from build123d import *

# Parameters (mm, degrees)
F0_R          = 28.5
F0_R_2        = 26.5
F1_DEPTH      = 1800
F2_R          = 5.25
F2_R_2        = 6
F3_DEPTH      = 28.501
F3_DEPTH_BACK = 28.501
F6_DEPTH      = 5
F7_R          = 5
F8_DEPTH      = 70
F11_DEPTH     = 5
F14_DEPTH     = 5


with BuildPart() as f1:
    # F0 (on Top) → F1 (new body)
    with BuildSketch(Plane.XY):
        Circle(F0_R)
        Circle(F0_R_2, mode=Mode.SUBTRACT)
    extrude(amount=F1_DEPTH)

    # F2 (on Front) → F3 (cut, two sides)
    with BuildSketch(Plane.XZ) as f3_sk:
        with Locations((0, 50)):
            Circle(F2_R)
        with Locations((0, 150)):
            Circle(F2_R)
        with Locations((0, 1420)):
            Circle(F2_R_2)
    extrude(amount=-F3_DEPTH, mode=Mode.SUBTRACT)
    extrude(f3_sk.sketch, amount=F3_DEPTH_BACK, mode=Mode.SUBTRACT)

    # F5 (on offset) → F6 (join)
    with BuildSketch(Plane.XZ.offset(28)):
        Polygon((-5, 41.3397459622), (5, 41.3397459622), (10, 50), (5, 58.6602540378), (-5, 58.6602540378), (-10, 50), align=None)
        Polygon((-5, 141.3397459622), (5, 141.3397459622), (10, 150), (5, 158.6602540378), (-5, 158.6602540378), (-10, 150), align=None)
    extrude(amount=F6_DEPTH)

    # F7 (on offset) → F8 (join)
    with BuildSketch(Plane.XZ.offset(28)):
        with Locations((0, 150)):
            Circle(F7_R)
        with Locations((0, 50)):
            Circle(F7_R)
    extrude(amount=-F8_DEPTH)

    # F10 (on offset) → F11 (join)
    with BuildSketch(Plane.XZ.offset(-28)):
        Polygon((-5, 141.3397459622), (5, 141.3397459622), (10, 150), (5, 158.6602540378), (-5, 158.6602540378), (-10, 150), align=None)
        Polygon((-5, 41.3397459622), (5, 41.3397459622), (10, 50), (5, 58.6602540378), (-5, 58.6602540378), (-10, 50), align=None)
    extrude(amount=-F11_DEPTH)

    # F13 (on offset) → F14 (join)
    with BuildSketch(Plane(origin=(0, 34, 0), x_dir=(-1, 0, 0), z_dir=(0, 1, 0))):
        Polygon((-10, 150), (-5, 141.3397459622), (5, 141.3397459622), (10, 150), (5, 158.6602540378), (-5, 158.6602540378), align=None)
        Polygon((-10, 50), (-5, 41.3397459622), (5, 41.3397459622), (10, 50), (5, 58.6602540378), (-5, 58.6602540378), align=None)
    extrude(amount=F14_DEPTH)


solid = f1.part
Design review of the part built by this model. Coordinates are the model's own, in mm. Coordinates: 2 decimals unless noted, no trailing zeros. Order: outer loops, then holes, each group sorted by start corner. A loop starts at its lowest first (then second) coordinate and runs counter-clockwise, first axis right, second up. Notation, with made-up numbers: (65, 28) -> (80, 28) arc R32 ccw to (80, 57) -> close; hole circle Ø1 at (68, 9). An arc over 180 degrees is marked (long way). One line per item, written item: value.
1) Clearance check with flat-ended pins moving along their axes: P1, Ø3, axis at x = 1.5, z = 1235, coming from the -Y side; P2, Ø8, axis at y = 13.5, z = 329, coming from the +X side; P3, Ø2.5, axis at x = -7, z = 48, coming from the +Y side. State where each tip first meets the part, or that it passes through.
Output values:
P1: stops at y = -28.5
P2: stops at x = 26.87
P3: stops at y = 39
2) We need section B-B, the plane z = 834. Give the boundary of the cut face in (x, y), then the cut area to 3 significant figures.
Output values:
outline: circle Ø57 at (0, 0); hole circle Ø53 at (0, 0)
area: 346 mm2
3) Draft analysis for pull direction X (two halves, no side actions). For faces 1 (the face through (19, -19, 0)), 2 (the face through (14.246, 22.345, 887.4)), state which applies: +X half, -X half, draft (parallel to the pull), parting line (faces both ways), or undercut.
Output values:
face 1: draft
face 2: undercut
4) To check wall thickness, follow probe 1 along Z at (x, y) = (0, -27); probe 2 along Z at (x, y) = (0, -26); probe 3 along X at (y, z) = (-0.5, 1331). State the ranges of each line that lie inside material, in increasing order. Write a range as [from, to].
Output values:
probe 1: z = [0, 44.75], [45, 55], [55.25, 144.75], [145, 155], [155.25, 1414], [1426, 1800]
probe 2: z = [45, 55], [145, 155]
probe 3: x = [-28.5, -26.5], [26.5, 28.5]
5) We need section A-A, the plane y = 13. Give the boundary of the cut face in (x, z), then the cut area to 3 significant figures.
Output values:
outline: (-25.36, 0) -> (-23.09, 0) -> (-23.09, 1800) -> (-25.36, 1800) -> close; circle Ø10 at (0, 50); circle Ø10 at (0, 150); (23.09, 0) -> (25.36, 0) -> (25.36, 1800) -> (23.09, 1800) -> close
area: 8,330 mm2
